Here's how the part is built. I have some questions about the finished solid (model axes, mm). A direction names the side the tool comes from. Round coordinates to 2 decimals unless told otherwise and drop trailing zeros. Write each loop counter-clockwise with the first axis right and the second up, starting at its lowest first coordinate (ties: lowest second). Pieces come first, ordered by that corner, then holes. Notation, with made-up numbers: M 52,14 L 98,14 A28 ccw 98,50 Z; hole C 36,73 d10. An arc over 180 degrees is marked long. Use one line per item in the form item = value. Start each with the question number.
Q1. For faces 5 (the face through (0, 1, 260)), 6 (the face through (80, -11, 58)), 7 (the face through (80, 14, 58)), which set-ups out of +Z, -Z, +X, -X, +Y, -Y let a thin tool reach every point of the face, with its end or its side?
Q2. We'd pull the mould along Y, two halves only. Please class faces 1 (the face through (-50, 20, 148)), 2 (the face through (80, -4, 108)), 3 (the face through (80, -8, 113)), 4 (the face through (-27, -5, 148)): +Y half, -Y half, draft (parallel to the pull), parting line (faces both ways), or undercut.
Q3. I'm going to push flat-ended pins straight in: pin 1 Ø5.5 at (x, y) = (78.5, -9) entering from -Z; pin 2 Ø5.5 at (x, y) = (90, -6) entering from +Z; pin 3 Ø6 at (y, z) = (7.5, 58.5) entering from +X. Where does each tip first touch, or does it pass through?
Q4. I need wall thicknesses on line 1 along X through (y, z) = (-15, 168.5); line 2 along Y through (x, z) = (56, 136); line 3 along X through (y, z) = (-10.5, 36). Which ranges of each line are inside material? Lowest first, please. Write a range as from..to.
Q5. I want a section at D-D on y = -17. List the corners of the cut face in (x, z) for me, and give its area (3 significant figures).
Q6. I want a section at B-B on x = -10. List the corners of the cut face in (y, z) for me, and give its area (3 significant figures).
Q7. I want a section at A-A on y = 0.5. List the corners of the cut face in (x, z) for me.
Q8. I want a section at C-C on z = 108.5. List the corners of the cut face in (x, y) for me, and give its area (3 significant figures).
```python
from build123d import *

# Parameters (mm, degrees)
F1_DEPTH = 300
F3_DEPTH = 25
F4_SIZE  = 2
F5_W     = 7
F5_H     = 10
F5_W_2   = 6
F6_DEPTH = 50


with BuildPart() as f1:
    # F0 (on Top) → F1 (new body)
    with BuildSketch(Plane.XY):
        with BuildLine():
            Line((-40, -5), (0, -5))
            Line((0, -5), (40, -5))
            ThreePointArc((40, -5), (43.535534, -6.464466), (45, -10))
            Line((45, -10), (45, -20))
            Line((45, -20), (55, -20))
            Line((55, -20), (55, 20))
            Line((55, 20), (45, 20))
            Line((45, 20), (45, 10))
            ThreePointArc((45, 10), (43.535534, 6.464466), (40, 5))
            Line((40, 5), (0, 5))
            Line((0, 5), (-40, 5))
            ThreePointArc((-40, 5), (-43.535534, 6.464466), (-45, 10))
            Line((-45, 10), (-45, 20))
            Line((-45, 20), (-55, 20))
            Line((-55, 20), (-55, -20))
            Line((-55, -20), (-45, -20))
            Line((-45, -20), (-45, -10))
            ThreePointArc((-45, -10), (-43.535534, -6.464466), (-40, -5))
        make_face()
    extrude(amount=F1_DEPTH)

    # F2 (on face) → F3 (cut)
    with BuildSketch(Plane(origin=(0, 5, 0), x_dir=(-1, 0, 0), z_dir=(0, 1, 0))):
        with BuildLine():
            ThreePointArc((-20, 45), (-18.535534, 41.464466), (-15, 40))
            Line((-15, 40), (15, 40))
            ThreePointArc((15, 40), (18.535534, 41.464466), (20, 45))
            Line((20, 45), (20, 255))
            ThreePointArc((20, 255), (18.535534, 258.535534), (15, 260))
            Line((15, 260), (-15, 260))
            ThreePointArc((-15, 260), (-18.535534, 258.535534), (-20, 255))
            Line((-20, 255), (-20, 45))
        make_face()
    extrude(amount=-F3_DEPTH, mode=Mode.SUBTRACT)

    # F4
    f4_edges = [f1.edges().sort_by_distance(p)[0] for p in [
        (0, -5, 260),
    ]]
    chamfer(f4_edges, length=F4_SIZE)

    # F5 (on face) → F6 (join)
    with BuildSketch(Plane.YZ.offset(55)):
        with Locations((-7.5, 283)):
            Rectangle(F5_W, F5_H)
        with Locations((17, 283)):
            Rectangle(F5_W_2, F5_H)
        with Locations((-7.5, 258)):
            Rectangle(F5_W, F5_H)
        with Locations((17, 258)):
            Rectangle(F5_W_2, F5_H)
        with Locations((-7.5, 233)):
            Rectangle(F5_W, F5_H)
        with Locations((17, 233)):
            Rectangle(F5_W_2, F5_H)
        with Locations((-7.5, 208)):
            Rectangle(F5_W, F5_H)
        with Locations((17, 208)):
            Rectangle(F5_W_2, F5_H)
        with Locations((-7.5, 183)):
            Rectangle(F5_W, F5_H)
        with Locations((17, 183)):
            Rectangle(F5_W_2, F5_H)
        with Locations((-7.5, 158)):
            Rectangle(F5_W, F5_H)
        with Locations((17, 158)):
            Rectangle(F5_W_2, F5_H)
        with Locations((-7.5, 133)):
            Rectangle(F5_W, F5_H)
        with Locations((17, 133)):
            Rectangle(F5_W_2, F5_H)
        with Locations((-7.5, 108)):
            Rectangle(F5_W, F5_H)
        with Locations((17, 108)):
            Rectangle(F5_W_2, F5_H)
        with Locations((-7.5, 83)):
            Rectangle(F5_W, F5_H)
        with Locations((17, 83)):
            Rectangle(F5_W_2, F5_H)
        with Locations((-7.5, 58)):
            Rectangle(F5_W, F5_H)
        with Locations((17, 58)):
            Rectangle(F5_W_2, F5_H)
        with Locations((-7.5, 33)):
            Rectangle(F5_W, F5_H)
        with Locations((17, 33)):
            Rectangle(F5_W_2, F5_H)
        with Locations((-7.5, 8)):
            Rectangle(F5_W, F5_H)
        with Locations((17, 8)):
            Rectangle(F5_W_2, F5_H)
    extrude(amount=F6_DEPTH)


solid = f1.part
```
Reported:
q1.face_5 = +Y, -Y
q1.face_6 = +Z, -Z, +X, -Y
q1.face_7 = +Z, -Z, +X
q2.face_1 = +Y half
q2.face_2 = undercut
q2.face_3 = draft
q2.face_4 = -Y half
q3.pin_1 = 3
q3.pin_2 = 288
q3.pin_3 = 55
q4.line_1 = -55..-45, 45..55
q4.line_2 = -11..-4, 14..20
q4.line_3 = -55..-45, 45..105
q5.outline = M -55,0 L -45,0 L -45,300 L -55,300 Z; M 45,0 L 55,0 L 55,300 L 45,300 Z
q5.area = 6,000 mm^2
q6.outline = M -5,0 L 5,0 L 5,40 L -3,40 L -5,38 Z; M -5,262 L -3,260 L 5,260 L 5,300 L -5,300 Z
q6.area = 796 mm^2
q7.outline = M -55,0 L 55,0 L 55,300 L -55,300 Z; hole M -20,45 A5 ccw -15,40 L 15,40 A5 ccw 20,45 L 20,255 A5 ccw 15,260 L -15,260 A5 ccw -20,255 Z
q8.outline = M -55,-20 L -45,-20 L -45,-10 A5 cw -40,-5 L -22,-5 L -20,-3 L -20,5 L -40,5 A5 cw -45,10 L -45,20 L -55,20 Z; M 20,-3 L 22,-5 L 40,-5 A5 cw 45,-10 L 45,-20 L 55,-20 L 55,-11 L 105,-11 L 105,-4 L 55,-4 L 55,14 L 105,14 L 105,20 L 45,20 L 45,10 A5 cw 40,5 L 20,5 Z
q8.area = 1,970 mm^2
